CAD build for the part. Positions are in the model's coordinates, mm. Face numbers are marked on the shaded views. A direction names the side the tool comes from. Give positions to 0.01 mm unless a question says otherwise; leave off trailing zeros. Order: outer loops, then holes, each group sorted by start corner. A loop starts at its lowest first (then second) coordinate and runs counter-clockwise, first axis right, second up.
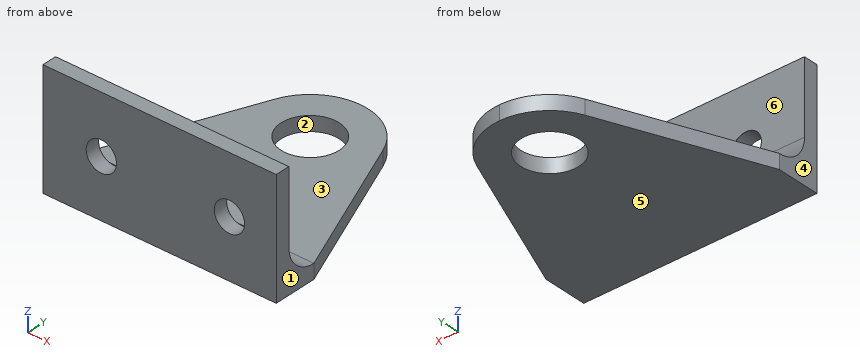
```python
from build123d import *

# Parameters (mm, degrees)
BOSS_EXTRUDE1_DEPTH           = 25.4
FILLET1_R                     = 6.35
M6_CLEARANCE_HOLE1_AT_2_COUNT = 2
M6_CLEARANCE_HOLE1_AT_2_PITCH = 27.890807904
SKETCH4_R                     = 6.35
CUT_EXTRUDE1_DEPTH            = 59.37764812


with BuildPart() as part:
    # Sketch1 → Boss-Extrude1 (new, symmetric)
    with BuildSketch(Plane(origin=(0, 0, 0), x_dir=(0, 0, -1), z_dir=(1, 0, 0))):
        Polygon((0, 0), (22.23, 0), (22.23, 47.63), (25.4, 47.63), (25.4, -3.17), (0, -3.17), align=None)
    extrude(amount=BOSS_EXTRUDE1_DEPTH, both=True)

    # Fillet1
    fillet1_edges = [part.edges().sort_by_distance(p)[0] for p in [
        (0, 0, -22.23),
    ]]
    fillet(fillet1_edges, radius=FILLET1_R)

    # Sketch3 → M6 Clearance Hole1 (revolve, cut)
    with BuildSketch(Plane(origin=(-12.7, 0, -12.7), x_dir=(0, 0, 1), z_dir=(1, 0, 0))):
        Polygon((0, 0), (0, 3.17), (3.3, 3.17), (3.3, 0.025), (3.325, 0), align=None)
    m6_clearance_hole1 = revolve(axis=Axis((-12.7, 6.35, -12.7), (0, -1, 0)), mode=Mode.SUBTRACT)

    # M6 Clearance Hole1 at 2: M6 Clearance Hole1 ×2
    with Locations(*[(i * M6_CLEARANCE_HOLE1_AT_2_PITCH, 0, 0) for i in range(1, M6_CLEARANCE_HOLE1_AT_2_COUNT)]):
        add(m6_clearance_hole1, mode=Mode.SUBTRACT)

    # Sketch4 → Cut-Extrude1 (cut, through all)
    with BuildSketch(Plane.XY.offset(-22.23)):
        with Locations((0, 34.93)):
            Circle(SKETCH4_R)
        with BuildLine():
            Line((25.4, 47.63), (-3e-08, 47.63))
            ThreePointArc((-3e-08, 47.63), (7.080670019, 45.472965052), (11.756103406, 39.734584552))
            Line((11.756103406, 39.734584552), (25.4, 6.35))
            Line((25.4, 6.35), (25.4, 47.63))
        make_face()
        with BuildLine():
            Line((-25.4, 47.63), (-25.4, 6.35))
            Line((-25.4, 6.35), (-11.756103406, 39.734584552))
            ThreePointArc((-11.756103406, 39.734584552), (-7.080670044, 45.472965035), (-3e-08, 47.63))
            Line((-3e-08, 47.63), (-25.4, 47.63))
        make_face()
    extrude(amount=-CUT_EXTRUDE1_DEPTH, mode=Mode.SUBTRACT)


solid = part.part
```
Item 1: Slice it at A-A (y = 37.5). Give the cut face in (x, z).
Item 2: Tool access for the marked faces 5 and 6: list every direction of +Z, -Z, +X, -X, +Y, -Y with a clear straight run to the whole face (end or side of a thin tool).
Item 3: Slice it at D-D (x = -20). Give the cut face in (y, z), and give its area (3 significant figures).
Item 4: Slice it at B-B (x = -12.7). Give the cut face in (y, z) (3 decimals), and give its area (3 significant figures).
Item 5: Two-plate mould, pull along X, no slides. Class the marked faces 1, 2, 3 and 4: released by +X, released by -X, zero draft, split by the parting line, or undercut.
Item 6: Drop flat-ended pins along their axis: pin 1 Ø8 at (x, y) = (-16, 27.5) entering from +Z; pin 2 Ø3 at (x, y) = (-20, 4) entering from +Z; pin 3 Ø1.5 at (x, z) = (9, -22.5) entering from +Y; pin 4 Ø8.5 at (x, z) = (15.19, -12.7) entering from -Y. Give the stop position or say it passes through.
Item 7: Wall check: L1, parallel to X at y = -0.85, z = -12.7; L2, parallel to Y at x = 0, z = -23.75; L3, parallel to Z at x = 12, y = 24. Give the ranges that are in metal, low to high.
Item 8: Slice it at C-C (z = -8). Give the cut face in (x, y).
A:
1. outline: (-12.67, -25.4) - (-5.81, -25.4) - (-5.81, -22.23) - (-12.67, -22.23) - close; (5.81, -25.4) - (12.67, -25.4) - (12.67, -22.23) - (5.81, -22.23) - close
2. face 5: -Z, +X, -X, +Y, -Y
2. face 6: +Z, +X, -X, +Y
3. outline: (-3.17, -25.4) - (19.56, -25.4) - (19.56, -22.23) - (6.35, -22.23) arc R6.35 cw to (0, -15.88) - (0, 0) - (-3.17, 0) - close
3. area: 151 mm2
4. outline: (-3.17, -25.4) - (37.425, -25.4) - (37.425, -22.23) - (6.35, -22.23) arc R6.35 cw to (0, -15.88) - (0, -16.025) - (-0.025, -16) - (-3.17, -16) - close; (-3.17, -9.4) - (-0.025, -9.4) - (0, -9.375) - (0, 0) - (-3.17, 0) - close
4. area: 187 mm2
5. face 1: released by +X
5. face 2: undercut
5. face 3: zero draft
5. face 4: released by -X
6. pin 1: stops at z = -22.23
6. pin 2: stops at z = -20.93
6. pin 3: stops at y = 44.59
6. pin 4: stops at y = -3.17
7. L1: x = -25.4 to -16, -9.4 to 11.89, 18.49 to 25.4
7. L2: y = -3.17 to 28.58, 41.28 to 47.63
7. L3: z = -25.4 to -22.23
8. outline: (-25.4, -3.17) - (25.4, -3.17) - (25.4, 0) - (-25.4, 0) - close
